Here's how the part is built. I have some questions about the finished solid (model axes, mm). A direction names the side the tool comes from. Round coordinates to 2 decimals unless told otherwise and drop trailing zeros. Order: outer loops, then holes, each group sorted by start corner. A loop starts at its lowest first (then second) coordinate and runs counter-clockwise, first axis right, second up. Notation, with made-up numbers: (31, -9.75) - (41, -9.75) arc R33 ccw to (41, 19.25) - close; hole circle Ø11 at (14, -23.75). An arc over 180 degrees is marked (long way). Answer as a JSON object with one key per item and string values.
```python
from build123d import *

# Parameters (mm, degrees)
F0_R     = 1.7182468223
F1_DEPTH = 304.8


with BuildPart() as f1:
    # F0 (on Front) → F1 (new body)
    with BuildSketch(Plane.XZ):
        with BuildLine():
            Line((-32.9967385804, 6.8048425582), (-28.4104094703, 49.945047138))
            ThreePointArc((-28.4104094703, 49.945047138), (-33.9877661328, 40.392821433), (-44.45, 36.8020574797))
            Line((-44.45, 36.8020574797), (-44.45, -1.302996767))
            ThreePointArc((-44.45, -1.302996767), (-37.7148079092, -4.0928046762), (-34.925, -10.827996767))
            Line((-34.925, -10.827996767), (-7.9375, -10.827996767))
            ThreePointArc((-7.9375, -10.827996767), (-5.6126600757, -5.2153366913), (0, -2.890496767))
            Line((0, -2.890496767), (-25.3759362201, -1.9807197434))
            ThreePointArc((-25.3759362201, -1.9807197434), (-31.0967184952, 0.7549521344), (-32.9967385804, 6.8048425582))
        make_face()
        with BuildLine():
            ThreePointArc((-44.45, 36.8020574797), (-54.883074079, 41.0682090736), (-59.8545699484, 51.1842020046))
            Line((-59.8545699484, 51.1842020046), (-53.9330768267, -11.720677504))
            ThreePointArc((-53.9330768267, -11.720677504), (-51.4937351249, -4.4161779541), (-44.45, -1.302996767))
            Line((-44.45, -1.302996767), (-44.45, 36.8020574797))
        make_face()
        with BuildLine():
            ThreePointArc((-44.45, -1.302996767), (-51.4937351249, -4.4161779541), (-53.9330768267, -11.720677504))
            ThreePointArc((-53.9330768267, -11.720677504), (-50.7345844929, -17.9854839484), (-44.1087293489, -20.3468811209))
            ThreePointArc((-44.1087293489, -20.3468811209), (-37.5952123318, -17.4414308994), (-34.925, -10.827996767))
            Line((-34.925, -10.827996767), (-41.275, -10.827996767))
            ThreePointArc((-41.275, -10.827996767), (-46.6950640303, -13.0730607973), (-44.45, -7.652996767))
            Line((-44.45, -7.652996767), (-44.45, -1.302996767))
        make_face()
        with BuildLine():
            ThreePointArc((-34.925, -10.827996767), (-37.7148079092, -4.0928046762), (-44.45, -1.302996767))
            Line((-44.45, -1.302996767), (-44.45, -7.652996767))
            ThreePointArc((-44.45, -7.652996767), (-42.2049359697, -8.5829327367), (-41.275, -10.827996767))
            Line((-41.275, -10.827996767), (-34.925, -10.827996767))
        make_face()
        with BuildLine():
            ThreePointArc((-34.925, -10.827996767), (-37.5952123318, -17.4414308994), (-44.1087293489, -20.3468811209))
            Line((-44.1087293489, -20.3468811209), (0, -18.765496767))
            ThreePointArc((0, -18.765496767), (-5.6126600757, -16.4406568427), (-7.9375, -10.827996767))
            Line((-7.9375, -10.827996767), (-34.925, -10.827996767))
        make_face()
        with BuildLine():
            ThreePointArc((-7.9375, -10.827996767), (-5.6126600757, -16.4406568427), (0, -18.765496767))
            ThreePointArc((0, -18.765496767), (5.6126600757, -16.4406568427), (7.9375, -10.827996767))
            ThreePointArc((7.9375, -10.827996767), (5.6126600757, -5.2153366913), (0, -2.890496767))
            ThreePointArc((0, -2.890496767), (-5.6126600757, -5.2153366913), (-7.9375, -10.827996767))
        make_face()
        with BuildLine():
            ThreePointArc((3.175, -10.827996767), (0, -14.002996767), (-3.175, -10.827996767))
            ThreePointArc((-3.175, -10.827996767), (0, -7.652996767), (3.175, -10.827996767))
        make_face(mode=Mode.SUBTRACT)
        with BuildLine():
            ThreePointArc((-28.1744419038, 52.672003233), (-28.2096407737, 53.7285661304), (-28.3150812936, 54.7804436962))
            ThreePointArc((-28.3150812936, 54.7804436962), (-33.74768808, 64.7504755351), (-44.45, 68.5419489863))
            Line((-44.45, 68.5419489863), (-44.45, 55.8216346736))
            ThreePointArc((-44.45, 55.8216346736), (-41.9507693419, 55.0544806154), (-40.8744419038, 52.672003233))
            ThreePointArc((-40.8744419038, 52.672003233), (-41.9507693419, 50.2895258506), (-44.45, 49.5223717924))
            Line((-44.45, 49.5223717924), (-44.45, 36.8020574797))
            ThreePointArc((-44.45, 36.8020574797), (-33.9877661328, 40.392821433), (-28.4104094703, 49.945047138))
            ThreePointArc((-28.4104094703, 49.945047138), (-28.2335438123, 51.3034300493), (-28.1744419038, 52.672003233))
        make_face()
        with BuildLine():
            Line((-44.45, 55.8216346736), (-44.45, 68.5419489863))
            ThreePointArc((-44.45, 68.5419489863), (-54.7455063411, 64.4027248883), (-59.8150941698, 54.532066035))
            ThreePointArc((-59.8150941698, 54.532066035), (-59.9233384244, 52.8591776278), (-59.8545699484, 51.1842020046))
            ThreePointArc((-59.8545699484, 51.1842020046), (-54.883074079, 41.0682090736), (-44.45, 36.8020574797))
            Line((-44.45, 36.8020574797), (-44.45, 49.5223717924))
            ThreePointArc((-44.45, 49.5223717924), (-47.2244419038, 52.672003233), (-44.45, 55.8216346736))
        make_face()
        with BuildLine():
            Line((-44.45, 68.5419489863), (-44.45, 93.947003233))
            ThreePointArc((-44.45, 93.947003233), (-51.5688441447, 97.1436793599), (-53.9093913596, 104.5880409142))
            Line((-53.9093913596, 104.5880409142), (-59.8150941698, 54.532066035))
            ThreePointArc((-59.8150941698, 54.532066035), (-54.7455063411, 64.4027248883), (-44.45, 68.5419489863))
        make_face()
        with Locations((-47.625, 88.994003233)):
            Circle(F0_R, mode=Mode.SUBTRACT)
        with BuildLine():
            ThreePointArc((-35.0093836339, 104.7370675109), (-34.9461193219, 104.1059409715), (-34.925, 103.472003233))
            ThreePointArc((-34.925, 103.472003233), (-37.7148079092, 96.7368111422), (-44.45, 93.947003233))
            Line((-44.45, 93.947003233), (-44.45, 68.5419489863))
            ThreePointArc((-44.45, 68.5419489863), (-33.74768808, 64.7504755351), (-28.3150812936, 54.7804436962))
            Line((-28.3150812936, 54.7804436962), (-35.0093836339, 104.7370675109))
        make_face()
        with BuildLine():
            ThreePointArc((-44.45, 93.947003233), (-37.7148079092, 96.7368111422), (-34.925, 103.472003233))
            ThreePointArc((-34.925, 103.472003233), (-34.9461193219, 104.1059409715), (-35.0093836339, 104.7370675109))
            ThreePointArc((-35.0093836339, 104.7370675109), (-44.5251023084, 112.9967071467), (-53.9093913596, 104.5880409142))
            ThreePointArc((-53.9093913596, 104.5880409142), (-51.5688441447, 97.1436793599), (-44.45, 93.947003233))
        make_face()
        with BuildLine():
            ThreePointArc((-41.275, 103.472003233), (-42.2049359697, 101.2269392027), (-44.45, 100.297003233))
            ThreePointArc((-44.45, 100.297003233), (-46.6950640303, 105.7170672633), (-41.275, 103.472003233))
        make_face(mode=Mode.SUBTRACT)
    extrude(amount=F1_DEPTH)


solid = f1.part
```
1. If I drill on L1, parallel to Z at x = -44, y = -131; L2, parallel to Z at x = -44.45, y = -104.5; L3, parallel to Z at x = -2, y = -202, over which ranges is the centre line in solid material (lowest first)? Write a range as [from, to].
Responses:
{"L1": "[-20.34, -13.97], [-7.69, 49.5], [55.85, 100.33], [106.61, 112.99]", "L2": "[-20.35, -14], [-7.65, 49.52], [55.82, 100.3], [106.65, 113]", "L3": "[-18.84, -13.29], [-8.36, -2.82]"}
2. Thinking about a two-plate mould opening in Z: for faces 1 (the face through (-42, -304.8, 32)), 2 (the face through (0.41, -150.27, -7.68)), 3 (the face through (-31.615, -150.266, 79.409)), which applies, pulls with the +Z half, pulls with the -Z half, needs draft (parallel to the pull), parting line crosses it, or undercut?
Responses:
{"face 1": "needs draft", "face 2": "undercut", "face 3": "pulls with the +Z half"}
3. For faces 4 (the face through (-30.736, -150.266, 28.073)), 5 (the face through (-42, 0, 32)), which set-ups out of +Z, -Z, +X, -X, +Y, -Y let a thin tool reach every point of the face, with its end or its side?
Responses:
{"face 4": "+X, +Y, -Y", "face 5": "+Z, -Z, +X, -X, +Y"}
4. Imagine slicing it at B-B (x = -16). List the corners of the cut face in (y, z) for me.
Responses:
{"outline": "(-304.8, -19.34) - (0, -19.34) - (0, -2.32) - (-304.8, -2.32) - close"}
5. For P1, Ø6, axis at y = -171.5, z = 39.5, coming from the -X side; P2, Ø5, axis at x = -39, y = -31, coming from the +Z side; P3, Ø12, axis at y = -214, z = 76.5, coming from the -X side, each with a flat end and sliding along its axis, tell me the tip position at first contact or that it passes through.
Responses:
{"P1": "x = -59.04", "P2": "z = 112.53", "P3": "x = -57.93"}
6. Imagine slicing it at A-A (y = -134). Give the number of separate pieces and of enclosed holes in the cut face, plus the area to 3 significant figures.
Responses:
{"separate pieces": "1", "enclosed holes": "5", "area": "3,800 mm2"}
7. Imagine slicing it at C-C (z = 65). List the corners of the cut face in (x, y) for me.
Responses:
{"outline": "(-58.58, -304.8) - (-29.68, -304.8) - (-29.68, 0) - (-58.58, 0) - close"}
